The listing builds one solid part. Answer for the finished solid, in the listing's coordinates (mm). Coordinates: 2 decimals unless noted, no trailing zeros. Loops run counter-clockwise (first coordinate to the right, second up) from the corner with the lowest first, then second, coordinate; pieces in that order, holes last. Notation, with made-up numbers: M -7,5.25 L 21,5.25 A9 ccw 21,20.25 Z; hole C -22.75,-32.5 d10. An arc over 180 degrees is marked long. Answer as a JSON object with one key per item and string values. Group by question number.
1. Given pin 1 (0.8 mm diameter, centred on x = -8.5, z = 1283.5, fed in from -Y), flat-ended and moving along its own axis, determine where the tip first touches the part or whether it passes through.
2. Straight lines are drawn through the part: L1, parallel to Y at x = -8, z = 1288.5; L2, parallel to Y at x = 8.5, z = 935. For each, find the intervals that lie inside material, in ascending order.
3. A cutting plane is placed at A-A on z = 1557. Give the vertices of the cut face in (x, y), and give its area (3 significant figures).
from build123d import *

# Parameters (mm, degrees)
BOSS_EXTRUDE1_DEPTH = 2000


with BuildPart() as part:
    # Sketch1 → Boss-Extrude1 (new body)
    with BuildSketch(Plane.XY):
        with BuildLine():
            Line((-8, -8.75), (8, -8.75))
            ThreePointArc((8, -8.75), (9.414213562, -8.164213562), (10, -6.75))
            Line((10, -6.75), (10, -3))
            ThreePointArc((10, -3), (9.707106781, -2.292893219), (9, -2))
            Line((9, -2), (8, -2))
            ThreePointArc((8, -2), (6, 0), (8, 2))
            Line((8, 2), (9, 2))
            ThreePointArc((9, 2), (9.707106781, 2.292893219), (10, 3))
            Line((10, 3), (10, 6.75))
            ThreePointArc((10, 6.75), (9.414213562, 8.164213562), (8, 8.75))
            Line((8, 8.75), (-8, 8.75))
            ThreePointArc((-8, 8.75), (-9.414213562, 8.164213562), (-10, 6.75))
            Line((-10, 6.75), (-10, 3))
            ThreePointArc((-10, 3), (-9.707106781, 2.292893219), (-9, 2))
            Line((-9, 2), (-8, 2))
            ThreePointArc((-8, 2), (-6, 0), (-8, -2))
            Line((-8, -2), (-9, -2))
            ThreePointArc((-9, -2), (-9.707106781, -2.292893219), (-10, -3))
            Line((-10, -3), (-10, -6.75))
            ThreePointArc((-10, -6.75), (-9.414213562, -8.164213562), (-8, -8.75))
        make_face()
    extrude(amount=BOSS_EXTRUDE1_DEPTH)


solid = part.part
From the geometry:
{
 "1": {"pin 1": "stops at y = -8.75"},
 "2": {"L1": "y = -8.75 to -2, 2 to 8.75", "L2": "y = -8.69 to -2, 2 to 8.69"},
 "3": {"outline": "M -10,-6.75 A2 ccw -8,-8.75 L 8,-8.75 A2 ccw 10,-6.75 L 10,-3 A1 ccw 9,-2 L 8,-2 A2 cw 8,2 L 9,2 A1 ccw 10,3 L 10,6.75 A2 ccw 8,8.75 L -8,8.75 A2 ccw -10,6.75 L -10,3 A1 ccw -9,2 L -8,2 A2 cw -8,-2 L -9,-2 A1 ccw -10,-3 Z", "area": "317 mm²"}
}
